Source: CAD feature listing. Evaluate the final solid. Frame: model axes, mm. A direction names the side the tool comes from. Give positions to 0.01 mm unless a question says otherwise; leave off trailing zeros. Order: outer loops, then holes, each group sorted by start corner. A loop starts at its lowest first (then second) coordinate and runs counter-clockwise, first axis right, second up. Notation, with made-up numbers: M 3.5,16 L 62.5,16 A11 cw 62.5,21 Z; hole C -13,44.5 d11. An arc over 180 degrees is marked long. Answer in a Markdown table with one row per item. Add a question column.
(1) Material intervals for line 1 along Z through (x, y) = (0, 9.25); line 2 along Y through (x, z) = (-23, -19); line 3 along Y through (x, z) = (-89.5, -71.5), sorted ascending.
(2) Section query D-D, the plane x = -14.5. Return loops of the section in (y, z), plus the area to 3 significant figures.
(3) Section query C-C, the plane z = 11. Return loops of the section in (x, y), plus the area to 3 significant figures.
(4) Section query A-A, the plane x = 0. Return loops of the section in (y, z).
(5) Section query B-B, the plane y = -15. Return loops of the section in (x, z).
(6) Mould query, pull axis Z, two halves, no side actions, for faces 3 (the face through (-95, -18.999, -24)), 4 (the face through (-55.966, -5.91, 2.157)), 5 (the face through (-58.262, -5.91, -50.656)). Classes: pulls with the +Z half, pulls with the -Z half, needs draft (parallel to the pull), parting line crosses it, or undercut.
(7) Set-up query: faces 1 (the face through (-95, 7.01, -24)), 2 (the face through (-100.8, -18.999, -64.5)). Return all of +Z, -Z, +X, -X, +Y, -Y with unobstructed straight access to the full face (end or side cutting, diameter ignored); none if empty.
(8) Pin query (flat end, axial travel): P1, Ø12, axis at x = -85, y = -6, coming from the +Z side; P2, Ø3, axis at x = -66, z = -11.5, coming from the -Y side; P3, Ø8, axis at x = 5, y = -6.5, coming from the +Z side. Return the tip coordinate at first contact, or that it passes through.
from build123d import *

# Parameters (mm, degrees)
F1_DEPTH      = 11.9888
F0_R          = 5.9944
F2_DEPTH      = 7.0104
F2_DEPTH_BACK = 18.9992
F0_R_2        = 13.0048
F3_DEPTH      = 14.0208
F3_DEPTH_BACK = 26.0096


with BuildPart() as f1:
    # F0 (on Front) → F1 (new body)
    with BuildSketch(Plane.XZ):
        with BuildLine():
            ThreePointArc((-102.9340252947, -19.0601129663), (-91.4840261862, -19.9144114295), (-85.9917, -29.9974))
            ThreePointArc((-85.9917, -29.9974), (-97.9932, -41.9989), (-109.9947, -29.9974))
            Line((-109.9947, -29.9974), (-109.9947, -70.0024))
            ThreePointArc((-109.9947, -70.0024), (-97.9932, -58.0009), (-85.9917, -70.0024))
            ThreePointArc((-85.9917, -70.0024), (-87.0411891719, -74.910501575), (-90.0061083773, -78.9602105395))
            Line((-90.0061083773, -78.9602105395), (-25.6162571026, -21.548007029))
            ThreePointArc((-25.6162571026, -21.548007029), (-19.305050019, -19.660505954), (-12.9493464286, -21.3922758668))
            ThreePointArc((-12.9493464286, -21.3922758668), (-24.9612819832, 1.4998138042), (-10.2946931272, 22.7889081157))
            Line((-10.2946931272, 22.7889081157), (-102.9340252947, -19.0601129663))
        make_face()
    extrude(amount=F1_DEPTH)

    # F0 (on Front) → F2 (join, two sides)
    with BuildSketch(Plane.XZ) as f2_sk:
        with BuildLine():
            ThreePointArc((-109.9947, -29.9974), (-97.9932, -41.9989), (-85.9917, -29.9974))
            ThreePointArc((-85.9917, -29.9974), (-91.4840261862, -19.9144114295), (-102.9340252947, -19.0601129663))
            ThreePointArc((-102.9340252947, -19.0601129663), (-108.0761885705, -23.4882261862), (-109.9947, -29.9974))
        make_face()
        with Locations((-97.9932, -29.9974)):
            Circle(F0_R, mode=Mode.SUBTRACT)
        with BuildLine():
            ThreePointArc((-85.9917, -70.0024), (-97.9932, -58.0009), (-109.9947, -70.0024))
            ThreePointArc((-109.9947, -70.0024), (-102.901301575, -80.9544108281), (-90.0061083773, -78.9602105395))
            ThreePointArc((-90.0061083773, -78.9602105395), (-87.0411891719, -74.910501575), (-85.9917, -70.0024))
        make_face()
        with Locations((-97.9932, -70.0024)):
            Circle(F0_R, mode=Mode.SUBTRACT)
    extrude(amount=-F2_DEPTH)
    extrude(f2_sk.sketch, amount=F2_DEPTH_BACK)

    # F0 (on Front) → F3 (join, two sides)
    with BuildSketch(Plane.XZ) as f3_sk:
        with BuildLine():
            ThreePointArc((25.0063, 0), (13.5625007824, 21.0088936457), (-10.2946931272, 22.7889081157))
            ThreePointArc((-10.2946931272, 22.7889081157), (-24.9612819832, 1.4998138042), (-12.9493464286, -21.3922758668))
            ThreePointArc((-12.9493464286, -21.3922758668), (12.2780250466, -21.7845160755), (25.0063, 0))
        make_face()
        Circle(F0_R_2, mode=Mode.SUBTRACT)
    extrude(amount=-F3_DEPTH)
    extrude(f3_sk.sketch, amount=F3_DEPTH_BACK)


solid = f1.part
Values follow:
| question | item | result |
|---|---|---|
| 1 | line 1 | z = -25.01 to -13, 13 to 25.01 |
| 1 | line 2 | y = -11.99 to 0 |
| 1 | line 3 | y = -19 to 7.01 |
| 2 | outline | M -26.01,-20.37 L -11.99,-20.37 L -11.99,-20.6 L 0,-20.6 L 0,-20.37 L 14.02,-20.37 L 14.02,20.37 L 0,20.37 L 0,20.89 L -11.99,20.89 L -11.99,20.37 L -26.01,20.37 Z |
| 2 | area | 1,640 mm² |
| 3 | outline | M -36.39,-11.99 L -22.46,-11.99 L -22.46,-26.01 L -6.94,-26.01 L -6.94,14.02 L -22.46,14.02 L -22.46,0 L -36.39,0 Z; M 6.94,-26.01 L 22.46,-26.01 L 22.46,14.02 L 6.94,14.02 Z |
| 3 | area | 1,410 mm² |
| 4 | outline | M -26.01,-25.01 L 14.02,-25.01 L 14.02,-13 L -26.01,-13 Z; M -26.01,13 L 14.02,13 L 14.02,25.01 L -26.01,25.01 Z |
| 5 | outline | C -97.99,-70 d24; C -97.99,-30 d24; C 0,0 d50.01; hole C -97.99,-70 d11.99; hole C -97.99,-30 d11.99; hole C 0,0 d26.01 |
| 6 | face 3 | needs draft |
| 6 | face 4 | pulls with the +Z half |
| 6 | face 5 | pulls with the -Z half |
| 7 | face 1 | +Z, -Z, -X, +Y |
| 7 | face 2 | +Z, -Z, +X, -X, -Y |
| 8 | P1 | stops at z = -8.25 |
| 8 | P2 | stops at y = -11.99 |
| 8 | P3 | stops at z = 24.99 |
